Design review of the part built by this model. Coordinates are the model's own, in mm. A direction names the side the tool comes from. Coordinates: 2 decimals unless noted, no trailing zeros. Order: outer loops, then holes, each group sorted by start corner. A loop starts at its lowest first (then second) coordinate and runs counter-clockwise, first axis right, second up. Notation, with made-up numbers: M -35.5,33 L 11.5,33 A16 cw 11.5,61 Z; hole C 53,61 d10. An arc over 180 degrees is marked long. Answer as a JSON object with one key per item and string values.
from build123d import *

# Parameters (mm, degrees)
BOSS_EXTRUDE7_START                  = 3.81
SKETCH31_W                           = 68.725
SKETCH31_H                           = 12.7
SKETCH31_W_2                         = 25.4
SKETCH31_H_2                         = 9.525
SKETCH31_W_3                         = 15.875
SKETCH31_H_3                         = 6.35
BOSS_EXTRUDE7_DEPTH                  = 12.7
M3_CLEARANCE_HOLE4_D                 = 3.2
CUT_EXTRUDE3_START                   = 6.35
CUT_EXTRUDE3_DEPTH                   = 3.175
CUT_EXTRUDE4_START                   = -6.35
CUT_EXTRUDE4_DEPTH                   = 3.175
BALL_START                           = 44.54897704
BALL_BALANCER_MASTER_MODEL_OUTLINE_R = 1.6
BALL_BALANCER_MASTER_MODEL_DEPTH     = 3.175


# Read off the part's stored shape, not the designer's step: Ball Balancer Master Model
with BuildPart() as part:
    # Sketch31 → Boss-Extrude7 (new body)
    # profile 1 of 2: a face of its own
    with BuildSketch(Plane(origin=(0, 9.162503731, 109.526818173), x_dir=(0, 0.9965191508346533, -0.08336415308621317), z_dir=(0, 0.08336415308621317, 0.9965191508346533)).offset(BOSS_EXTRUDE7_START)):
        with Locations((13.36147704, 0)):
            Rectangle(SKETCH31_W, SKETCH31_H)
        with Locations((31.84897704, 0)):
            Rectangle(SKETCH31_W_2, SKETCH31_H_2, mode=Mode.SUBTRACT)
    # profile 2 of 2: a face of its own
    with BuildSketch(Plane(origin=(0, 9.162503731, 109.526818173), x_dir=(0, 0.9965191508346533, -0.08336415308621317), z_dir=(0, 0.08336415308621317, 0.9965191508346533)).offset(BOSS_EXTRUDE7_START)):
        with Locations((-28.93852296, 0)):
            Rectangle(SKETCH31_W_3, SKETCH31_H_3)
    extrude(amount=-BOSS_EXTRUDE7_DEPTH)

    # M3 Clearance Hole4 (through all)
    with Locations(Plane.ZY.offset(3.175)):
        with Locations((-85.094578454, 48.544265488), (109.540435581, -21.469007696)):
            Hole(M3_CLEARANCE_HOLE4_D / 2)

    # Sketch35 → Cut-Extrude3 (cut)
    with BuildSketch(Plane.ZY.offset(CUT_EXTRUDE3_START)):
        Polygon((108.746392023, -11.977162785), (102.225823269, -10.203359146), (102.418495416, -12.506525157), align=None)
    extrude(amount=-CUT_EXTRUDE3_DEPTH, mode=Mode.SUBTRACT)

    # Sketch36 → Cut-Extrude4 (cut)
    with BuildSketch(Plane.ZY.offset(CUT_EXTRUDE4_START)):
        Polygon((102.225823269, -10.203359146), (108.746392023, -11.977162785), (102.418495416, -12.506525157), align=None)
    extrude(amount=CUT_EXTRUDE4_DEPTH, mode=Mode.SUBTRACT)

    # Ball Balancer Master Model outline → Ball Balancer Master Model (cut)
    with BuildSketch(Plane(origin=(0, 0, 0), x_dir=(1, 0, 0), z_dir=(0, 0.9965191508346533, -0.08336415308621321)).offset(BALL_START)):
        with Locations((0, -107.369396203)):
            Circle(BALL_BALANCER_MASTER_MODEL_OUTLINE_R)
    extrude(amount=BALL_BALANCER_MASTER_MODEL_DEPTH, mode=Mode.SUBTRACT)


solid = part.part
1) To check wall thickness, follow L1, parallel to X at y = 49.5, z = 100.75; L2, parallel to Y at x = -0.25, z = 110.25; L3, parallel to Y at x = 3, z = 106.5. State the ranges of each line that lie inside material, in increasing order.
Taken from the geometry:
{"L1": "x = -6.35 to -4.76, 4.76 to 6.35", "L2": "y = -27.78 to -22.9, -20.03 to 28.44", "L3": "y = -28.1 to 28.13, 53.61 to 56.8"}
2) Add section B-B (x = 5.5). State the section outline as (y, z) points, and give its area (3 significant figures).
Taken from the geometry:
{"outline": "M -11.98,108.75 L -10.2,102.23 L 55.98,96.69 L 57.04,109.35 L -11.45,115.07 Z", "area": "865 mm2"}
3) Mouldability with a two-part tool opening along Z and no side actions: class faces 6 (the flat face through (-4.785, -11.103, 105.532)), 7 (the cylindrical face through (0.04, -22.44, 110.81)), 8 (the flat face through (-0.99, 53.47, 104.78)) as released by +Z, released by -Z, zero draft, split by the parting line, or undercut.
Taken from the geometry:
{"face 6": "released by -Z", "face 7": "undercut", "face 8": "released by +Z"}
4) Tool access review of faces 1 (the flat face through (-4.74, -11.71, 111.95)), 2 (the flat face through (0.04, -27.79, 110.16)), 3 (the flat face through (4.78, -11.71, 111.95)), 4 (the flat face through (0, 28, 105)), 5 (the flat face through (4.785, -11.078, 105.44)): name each direction out of +Z, -Z, +X, -X, +Y, -Y from which nothing blocks a thin tool from reaching the whole face with its end or side.
Taken from the geometry:
{"face 1": "+Z, -X, -Y", "face 2": "+Z, +X, -X, -Y", "face 3": "+Z, +X, -Y", "face 4": "-Z", "face 5": "-Z, +X, -Y"}
5) Add section C-C (y = 18.5). State the section outline as (x, z) points.
Taken from the geometry:
{"outline": "M -6.35,99.82 L 6.35,99.82 L 6.35,112.57 L -6.35,112.57 Z"}
6) Add section A-A (y = 32.5). State the section outline as (x, z) points, and give its area (3 significant figures).
Taken from the geometry:
{"outline": "M -6.35,98.65 L -4.76,98.65 L -4.76,111.4 L -6.35,111.4 Z; M 4.76,98.65 L 6.35,98.65 L 6.35,111.4 L 4.76,111.4 Z", "area": "40.5 mm2"}
7) Insertion check: pin 1 Ø5 at (y, z) = (-21.47, 109.54) entering from +X (3 decimals); pin 2 Ø4 at (x, z) = (-2.5, 109.5) entering from -Y; pin 3 Ø1 at (x, z) = (-3, 105) entering from +Y. Each pin has a flat end and moves straight along its axis. Give the tip position at first contact, or say it passes through.
Taken from the geometry:
{"pin 1": "stops at x = 3.175", "pin 2": "stops at y = -28.01", "pin 3": "stops at y = 56.72"}
